Could you check a few things on this model? Use its own coordinates, in mm. Face numbers are marked on the shaded views. Coordinates: 2 decimals unless noted, no trailing zeros. Loops run counter-clockwise (first coordinate to the right, second up) from the corner with the lowest first, then second, coordinate; pieces in that order, holes last. Notation, with made-up numbers: M 49.5,18 L 54.5,18 A15 cw 54.5,42 Z; hole C 51,68 d11. An arc over 180 degrees is marked long. Write each question's results on one line, items separated by ' | '.
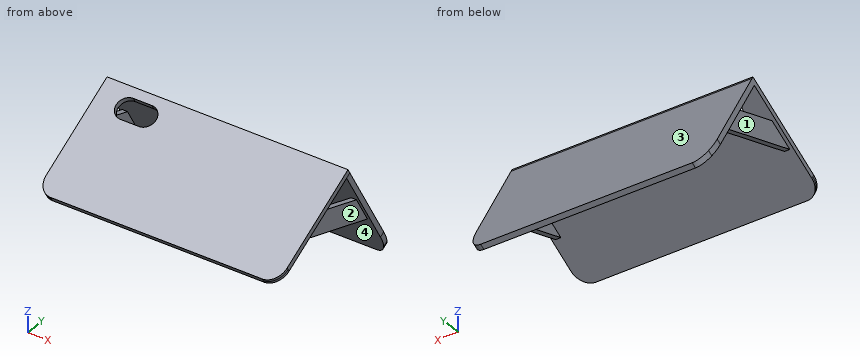
```python
from build123d import *

# Parameters (mm, degrees)
EXTRUDE012_DEPTH                          = 2
EXTRUDE013_DEPTH                          = 2
EXTRUDE014_DEPTH                          = 2
EXTRUDE011_DEPTH                          = 1
EXTRUDE011_ONTO_SKETCH012_PLACEMENT_ANGLE = 210


with BuildPart() as extrude012:
    # Facebinder001 → Extrude012 (new body)
    with BuildSketch(Plane(origin=(0, 18.8977675755, 30.9501387124), x_dir=(-1, 0, 0), z_dir=(0, -0.8660254038, -0.5))):
        with BuildLine():
            Line((-45.25, 13.204464849), (-45.25, -23.9452774122))
            Line((-45.25, -23.9452774122), (45.25, -23.9452774122))
            Line((45.25, -23.9452774122), (45.25, 13.2044648491))
            add(Edge.make_bspline(
                [(44.2347028524, 19.5723342968), (45.25, 16.7121588166), (45.25, 13.2044648491)],
                knots=[0.953420723, 0.953420723, 0.953420723, 1.5707963268, 1.5707963268, 1.5707963268], degree=2, weights=[1, 0.9527330472, 1]))
            add(Edge.make_bspline(
                [(39.75, 24.204464849), (42.590402015, 24.204464849), (44.2347028524, 19.5723342968)],
                knots=[0, 0, 0, 0.953420723, 0.953420723, 0.953420723], degree=2, weights=[1, 0.8885092072, 1]))
            Line((39.75, 24.204464849), (-39.75, 24.204464849))
            add(Edge.make_bspline(
                [(-44.2347028524, 19.5723342968), (-42.590402015, 24.204464849), (-39.75, 24.204464849)],
                knots=[5.3297645842, 5.3297645842, 5.3297645842, 6.2831853072, 6.2831853072, 6.2831853072], degree=2, weights=[1, 0.8885092072, 1]))
            add(Edge.make_bspline(
                [(-45.25, 13.204464849), (-45.25, 16.7121588165), (-44.2347028524, 19.5723342968)],
                knots=[4.7123889804, 4.7123889804, 4.7123889804, 5.3297645842, 5.3297645842, 5.3297645842], degree=2, weights=[1, 0.9527330472, 1]))
        make_face()
    extrude(amount=EXTRUDE012_DEPTH)


with BuildPart() as extrude013:
    # Sketch013 → Extrude013 (new body)
    with BuildSketch(Plane.YZ.offset(44)):
        Polygon((-15.020984158, 37.8620624495), (18.5712846291, 27.5156237634), (12.6930780618, 37.6969761952), (-5.5661322003, 43.3208237725), align=None)
    extrude(amount=-EXTRUDE013_DEPTH)


with BuildPart() as extrude014:
    # Sketch013 → Extrude014 (new body)
    with BuildSketch(Plane.YZ.offset(44)):
        Polygon((-15.020984158, 37.8620624495), (18.5712846291, 27.5156237634), (12.6930780618, 37.6969761952), (-5.5661322003, 43.3208237725), align=None)
    extrude(amount=EXTRUDE014_DEPTH)


with BuildPart() as extrude014_1:
    # Extrude014 placement: moved
    add(extrude014.part.moved(Location((-88, 0, 0))))


with BuildPart() as connect003:
    # Sketch012 as drawn → Extrude011 (new, symmetric)
    with BuildSketch(Plane.XY):
        with BuildLine():
            add(Edge.make_bspline(
                [(-39.7453392309, 11.9568462189), (-45.2533288617, 11.9676394264), (-45.25, 5.6081389921)],
                knots=[6.2710703316, 6.2710703316, 6.2710703316, 7.8406972721, 7.8406972721, 7.8406972721], degree=2, weights=[1, 0.7075201008, 1]))
            Line((-45.25, 5.6081389921), (-45.25, -31.84))
            Line((-45.25, -31.84), (45.2563247467, -31.84))
            Line((45.2563247467, -31.84), (45.2563247467, 5.6002976112))
            add(Edge.make_bspline(
                [(45.2563247467, 5.6002976112), (45.2564552158, 11.9567126485), (39.75, 11.9568462189)],
                knots=[4.7124493405, 4.7124493405, 4.7124493405, 6.2832273717, 6.2832273717, 6.2832273717], degree=2, weights=[1, 0.7071132496, 1]))
            Line((39.75, 11.9568462189), (-39.7453392309, 11.9568462189))
        make_face()
        with BuildLine():
            ThreePointArc((-26.25, -28.34), (-22.25, -24.34), (-26.25, -20.34))
            Line((-26.25, -20.34), (-33.25, -20.34))
            ThreePointArc((-33.25, -20.34), (-37.25, -24.34), (-33.25, -28.34))
            Line((-33.25, -28.34), (-26.25, -28.34))
        make_face(mode=Mode.SUBTRACT)
    extrude(amount=EXTRUDE011_DEPTH, both=True)


with BuildPart() as connect003_1:
    # Extrude011 onto Sketch012 placement: moved
    add(connect003.part.moved(Location((0, -20.65, 35.7668491763))).rotate(Axis((0, -20.65, 35.7668491763), (1, 0, 0)), EXTRUDE011_ONTO_SKETCH012_PLACEMENT_ANGLE))

    # Connect003: union Extrude012, Extrude013, Extrude014
    add(extrude012.part)
    add(extrude013.part)
    add(extrude014_1.part)


solid = connect003_1.part
```
(1) Will these pins go through, and if not, where does the flat tip stop? P1, Ø2, axis at x = -8.5, z = 37, coming from the -Y side; P2, Ø1, axis at x = -20, z = 40, coming from the -Y side; P3, Ø6, axis at x = -4.5, y = 14.5, coming from the -Z side.
Reported:
P1: stops at y = -22.25 | P2: stops at y = -16.18 | P3: stops at z = 29.37
(2) Imagine slicing it at C-C, the plane z = 36.5. List the corners of the cut face in (x, y) for me.
Reported:
outline: M -45.25,-21.38 L 45.26,-21.38 L 45.26,-17.38 L -45.25,-17.38 Z; M -45.25,13.38 L -44,13.38 L -44,-10.6 L -42,-10.6 L -42,13.38 L 42,13.38 L 42,-10.6 L 44,-10.6 L 44,13.38 L 45.25,13.38 L 45.25,15.69 L -45.25,15.69 Z
(3) If we mould it in two halves opening along X, with no side actions, what happens to the marked faces 1, 2, 3 and 4? For each: released by +X, released by -X, zero draft, split by the parting line, or undercut.
Reported:
face 1: released by -X | face 2: released by +X | face 3: zero draft | face 4: undercut
(4) Imagine slicing it at B-B, the plane y = 9. List the corners of the cut face in (x, z) for me, and give its area (3 significant figures).
Reported:
outline: M -45.25,44.09 L 45.25,44.09 L 45.25,48.09 L -45.25,48.09 Z; M -44,30.46 L -42,30.46 L -42,38.83 L -44,38.83 Z; M 42,30.46 L 44,30.46 L 44,38.83 L 42,38.83 Z | area: 395 mm2
(5) Please list where these lines run through material, in increasing order: probe 1 along X at (y, z) = (0.5, 47); probe 2 along Y at (x, z) = (-1.5, 43.5); probe 3 along Y at (x, z) = (25.5, 31). Write a range as from..to.
Reported:
probe 1: x = -45.25..-37.23, -22.27..45.26 | probe 2: y = -9.26..-5.26, 9.34..11.65 | probe 3: y = -30.91..-26.91, 16.56..18.87
